The listing builds one solid part. Answer for the finished solid, in the listing's coordinates (mm). Face numbers are marked on the shaded views. A direction names the side the tool comes from. Round coordinates to 2 decimals unless told otherwise and drop trailing zeros. Write each loop counter-clockwise with the first axis right and the second up, starting at its lowest first coordinate (ties: lowest second). Pieces come first, ordered by that corner, then holes. Notation, with made-up numbers: (-25.75, -1.75) - (15.25, -1.75) arc R6 cw to (15.25, 8.25) - close; hole circle Ø10 at (-9.75, 29.25). An arc over 180 degrees is marked (long way). Answer in a Markdown table with one row per item.
from build123d import *

# Parameters (mm, degrees)
SKETCH1_W           = 40
SKETCH1_H           = 20
BOSS_EXTRUDE1_DEPTH = 40
SKETCH2_R           = 1.5
BOSS_EXTRUDE2_DEPTH = 8
SKETCH4_W           = 8
SKETCH4_H           = 40
SKETCH4_W_2         = 40
SKETCH4_H_2         = 8
BOSS_EXTRUDE4_DEPTH = 3
FILLET1_R           = 2
SKETCH6_W           = 7
SKETCH6_H           = 20
BOSS_EXTRUDE5_DEPTH = 1


with BuildPart() as part:
    # Sketch1 → Boss-Extrude1 (new body)
    with BuildSketch(Plane.XY):
        with Locations((20, 10)):
            Rectangle(SKETCH1_W, SKETCH1_H)
    extrude(amount=BOSS_EXTRUDE1_DEPTH)

    # Sketch2 → Boss-Extrude2 (add)
    with BuildSketch(Plane(origin=(40, 0, 0), x_dir=(0, 0, -1), z_dir=(1, 0, 0))):
        with Locations(Location((-10, 10, 0), (0, 0, 180))):
            Circle(SKETCH2_R)
    extrude(amount=BOSS_EXTRUDE2_DEPTH)

    # Sketch4 → Boss-Extrude4 (add)
    with BuildSketch(Plane(origin=(48, 0, 0), x_dir=(0, 0, -1), z_dir=(1, 0, 0))):
        with Locations((-10, 10)):
            Rectangle(SKETCH4_W, SKETCH4_H)
        with Locations((-10, 10)):
            Rectangle(SKETCH4_W_2, SKETCH4_H_2)
    extrude(amount=BOSS_EXTRUDE4_DEPTH)

    # Fillet1
    fillet1_edges = [part.edges().sort_by_distance(p)[0] for p in [
        (49.5, 14, 30),
        (49.5, 6, 14),
        (49.5, 6, 30),
        (49.5, 6, -10),
        (49.5, 14, 6),
        (49.5, 14, -10),
        (49.5, 30, 6),
        (49.5, 14, 14),
        (49.5, 30, 14),
        (49.5, -10, 14),
        (49.5, 6, 6),
        (49.5, -10, 6),
    ]]
    fillet(fillet1_edges, radius=FILLET1_R)

    # Sketch6 → Boss-Extrude5 (add)
    with BuildSketch(Plane(origin=(34, 0, 0), x_dir=(0, 0, -1), z_dir=(1, 0, 0))):
        with Locations((-43.5, 10)):
            Rectangle(SKETCH6_W, SKETCH6_H)
        with Locations((3.5, 10)):
            Rectangle(SKETCH6_W, SKETCH6_H)
    extrude(amount=BOSS_EXTRUDE5_DEPTH)


solid = part.part
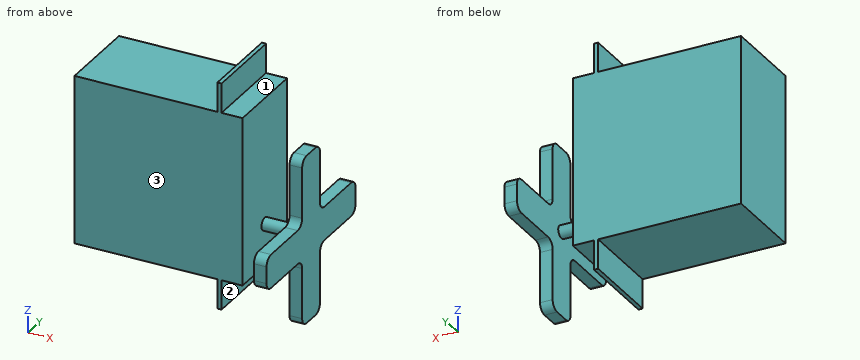
(1) Section D-D (x = 46) is taken. Give the vertices of the cut face in (y, z), and give its area (3 significant figures).
Checked values:
| item | result |
|---|---|
| outline | circle Ø3 at (10, 10) |
| area | 7.07 mm2 |
(2) Section B-B (y = 10) is taken. Give the vertices of the cut face in (x, z), and give its area (3 significant figures).
Checked values:
| item | result |
|---|---|
| outline | (0, 0) - (34, 0) - (34, -7) - (35, -7) - (35, 0) - (40, 0) - (40, 8.5) - (48, 8.5) - (48, -10) - (51, -10) - (51, 30) - (48, 30) - (48, 11.5) - (40, 11.5) - (40, 40) - (35, 40) - (35, 47) - (34, 47) - (34, 40) - (0, 40) - close |
| area | 1,760 mm2 |
(3) Find the intervals of material crossed by line 1 (X direction, y = 10, z = 20.5); line 2 (X direction, y = 26, z = 8); line 3 (X direction, y = 7, z = 34.5), in increasing order.
Checked values:
| item | result |
|---|---|
| line 1 | x = 0 to 40, 48 to 51 |
| line 2 | x = 48 to 51 |
| line 3 | x = 0 to 40 |
(4) Section A-A (z = 17) is taken. Give the vertices of the cut face in (x, y), and give its area (3 significant figures).
Checked values:
| item | result |
|---|---|
| outline | (0, 0) - (40, 0) - (40, 20) - (0, 20) - close; (48, 6) - (51, 6) - (51, 14) - (48, 14) - close |
| area | 824 mm2 |
(5) Section C-C (z = 10) is taken. Give the vertices of the cut face in (x, y).
Checked values:
| item | result |
|---|---|
| outline | (0, 0) - (40, 0) - (40, 8.5) - (48, 8.5) - (48, -10) - (51, -10) - (51, 30) - (48, 30) - (48, 11.5) - (40, 11.5) - (40, 20) - (0, 20) - close |
(6) Flat-ended cylindrical pins translate along their axes: pin 1 (5.5 mm diameter, centred on x = 37.5, y = 6, fed in from -Z); pin 2 (1.5 mm diameter, centred on x = 49.5, y = 23.5, fed in from -Z); pin 3 (5.5 mm diameter, centred on y = 8.5, z = 42, fed in from +X). Find the tip coordinate at first contact, or state that the pin passes through.
Checked values:
| item | result |
|---|---|
| pin 1 | stops at z = -7 |
| pin 2 | stops at z = 6 |
| pin 3 | stops at x = 40 |
(7) For the marked faces 1, 2 and 3, determine the directions among +Z, -Z, +X, -X, +Y, -Y from which every point of the face is accessible in a straight line to the end or side of a thin tool.
Checked values:
| item | result |
|---|---|
| face 1 | +Z, +X, +Y, -Y |
| face 2 | -Z, +Y, -Y |
| face 3 | +Z, -Z, -X, -Y |
